```python
from build123d import *

# Parameters (mm, degrees)
F2_DEPTH   = 3.175
F1_R       = 3.3099800026
F2_FACE_R  = 15.875
F3_DEPTH   = 3.176
F4_DEPTH   = 3.176
F5_DEPTH   = 3.176
F1_W       = 6.5204764251
F1_H       = 1.0553477332
F6_DEPTH   = 3.429
F7_DEPTH   = 3.175
F8_DEPTH   = 3.175
F10_DEPTH  = 3.175
F1_R_2     = 1.2371702014
F10_FACE_R = 3.3099800026
F10_FACE_W = 6.5204764251
F10_FACE_H = 1.0553477332
F11_DEPTH  = 3.43
F12_DEPTH  = 3.429


with BuildPart() as f2:
    # F0 (on Front) → F2 (new body)
    with BuildSketch(Plane.XZ):
        with BuildLine():
            ThreePointArc((-15.3480242567, 4.0563254821), (-2.0452065819, -15.7427048196), (15.875, 0))
            ThreePointArc((15.875, 0), (15.3869963752, 3.9058888297), (13.9529883401, 7.5716406003))
            ThreePointArc((13.9529883401, 7.5716406003), (12.6412349384, 9.6028539629), (11.0362168136, 11.4112901743))
            ThreePointArc((11.0362168136, 11.4112901743), (9.0476421038, 13.0443779983), (6.8213515593, 14.3347405943))
            ThreePointArc((6.8213515593, 14.3347405943), (5.0774604505, 15.0411110086), (3.2622452096, 15.5361958404))
            ThreePointArc((3.2622452096, 15.5361958404), (1.6398957334, 15.7900717853), (0, 15.875))
            ThreePointArc((0, 15.875), (-2.3954258199, 15.693232941), (-4.7359968989, 15.152094191))
            ThreePointArc((-4.7359968989, 15.152094191), (-6.342661706, 14.552878323), (-7.8753225223, 13.7838644861))
            ThreePointArc((-7.8753225223, 13.7838644861), (-9.4847902105, 12.730058117), (-10.9549720741, 11.4893085891))
            ThreePointArc((-10.9549720741, 11.4893085891), (-13.6665362642, 8.0772155808), (-15.3480242567, 4.0563254821))
        make_face()
    extrude(amount=F2_DEPTH)

    # F1 (on face) + F2_face (on face) → F3 (cut, through all)
    with BuildSketch(Plane.XZ):
        with Locations((-6.1555983319, 4.3306481437)):
            Circle(F1_R)
    with BuildSketch(Plane.XZ.offset(3.175)):
        Circle(F2_FACE_R)
    extrude(amount=F3_DEPTH, mode=Mode.SUBTRACT)

    # F1 (on face) → F4 (cut, through all)
    with BuildSketch(Plane.XZ):
        with Locations((6.1544640741, 4.4018082744)):
            Circle(F1_R)
    extrude(amount=F4_DEPTH, mode=Mode.SUBTRACT)

    # F1 (on face) → F5 (cut, through all)
    with BuildSketch(Plane.XZ):
        with BuildLine():
            Line((13.2357986914, 0.0787362223), (-13.2809156822, 0.0787362223))
            ThreePointArc((-13.2809156822, 0.0787362223), (-0.0225584954, -11.1437029045), (13.2357986914, 0.0787362223))
        make_face()
    extrude(amount=F5_DEPTH, mode=Mode.SUBTRACT)

    # F1 (on face) → F6 (join)
    with BuildSketch(Plane.XZ):
        with Locations((6.1458884738, 9.15713422)):
            Rectangle(F1_W, F1_H)
    extrude(amount=F6_DEPTH)

    # F0 (on Front) → F7 (join)
    with BuildSketch(Plane.XZ):
        with BuildLine():
            Line((-11.9195533916, 18.9222916961), (-15.3480242567, 4.0563254821))
            ThreePointArc((-15.3480242567, 4.0563254821), (-13.6665362642, 8.0772155808), (-10.9549720741, 11.4893085891))
            Line((-10.9549720741, 11.4893085891), (-11.9195533916, 18.9222916961))
        make_face()
    extrude(amount=F7_DEPTH)

    # F0 (on Front) → F8 (join)
    with BuildSketch(Plane.XZ):
        with BuildLine():
            Line((-7.8753225223, 24.8427737317), (-10.9549720741, 11.4893085891))
            ThreePointArc((-10.9549720741, 11.4893085891), (-9.4847902105, 12.730058117), (-7.8753225223, 13.7838644861))
            Line((-7.8753225223, 13.7838644861), (-7.8753225223, 24.8427737317))
        make_face()
    extrude(amount=F8_DEPTH)

    # F0 (on Front) → F10 (join)
    with BuildSketch(Plane.XZ):
        with BuildLine():
            Line((0, 29.9478769302), (-4.7359968989, 15.152094191))
            ThreePointArc((-4.7359968989, 15.152094191), (-2.3954258199, 15.693232941), (0, 15.875))
            Line((0, 15.875), (0, 29.9478769302))
        make_face()
        with BuildLine():
            ThreePointArc((0, 15.875), (1.6398957334, 15.7900717853), (3.2622452096, 15.5361958404))
            Line((3.2622452096, 15.5361958404), (3.2622452096, 30.0202061216))
            Line((3.2622452096, 30.0202061216), (0, 15.875))
        make_face()
        with BuildLine():
            ThreePointArc((3.2622452096, 15.5361958404), (5.0774604505, 15.0411110086), (6.8213515593, 14.3347405943))
            Line((6.8213515593, 14.3347405943), (9.8336311057, 27.3960871034))
            Line((9.8336311057, 27.3960871034), (3.2622452096, 15.5361958404))
        make_face()
        with BuildLine():
            ThreePointArc((6.8213515593, 14.3347405943), (9.0476421038, 13.0443779983), (11.0362168136, 11.4112901743))
            Line((11.0362168136, 11.4112901743), (14.0054738149, 24.286089465))
            Line((14.0054738149, 24.286089465), (6.8213515593, 14.3347405943))
        make_face()
        with BuildLine():
            ThreePointArc((11.0362168136, 11.4112901743), (12.6412349384, 9.6028539629), (13.9529883401, 7.5716406003))
            Line((13.9529883401, 7.5716406003), (17.5813417882, 19.8162570596))
            Line((17.5813417882, 19.8162570596), (11.0362168136, 11.4112901743))
        make_face()
        with BuildLine():
            Line((-4.7359968989, 27.3960871034), (-7.8753225223, 13.7838644861))
            ThreePointArc((-7.8753225223, 13.7838644861), (-6.342661706, 14.552878323), (-4.7359968989, 15.152094191))
            Line((-4.7359968989, 15.152094191), (-4.7359968989, 27.3960871034))
        make_face()
    extrude(amount=F10_DEPTH)

    # F1 (on face) + F10_face (on face) → F11 (cut, through all)
    with BuildSketch(Plane.XZ):
        with Locations((-12.1244213607, 7.7306859973)):
            Circle(F1_R_2)
    with BuildSketch(Plane(origin=(0.4916351087, -3.175, 5.8381828157), x_dir=(1, 0, 0), z_dir=(0, -1, 0))):
        with BuildLine():
            ThreePointArc((-15.8396593653, -1.7818573336), (-2.5368416906, -21.5808876353), (15.3833648913, -5.8381828157))
            ThreePointArc((15.3833648913, -5.8381828157), (14.8953612665, -1.932293986), (13.4613532315, 1.7334577846))
            Line((13.4613532315, 1.7334577846), (17.0897066795, 13.9780742439))
            Line((17.0897066795, 13.9780742439), (10.544581705, 5.5731073586))
            Line((10.544581705, 5.5731073586), (13.5138387063, 18.4479066493))
            Line((13.5138387063, 18.4479066493), (6.3297164506, 8.4965577786))
            Line((6.3297164506, 8.4965577786), (9.3419959971, 21.5579042877))
            Line((9.3419959971, 21.5579042877), (2.770610101, 9.6980130247))
            Line((2.770610101, 9.6980130247), (2.770610101, 24.1820233059))
            Line((2.770610101, 24.1820233059), (-0.4916351087, 10.0368171843))
            Line((-0.4916351087, 10.0368171843), (-0.4916351087, 24.1096941145))
            Line((-0.4916351087, 24.1096941145), (-5.2276320076, 9.3139113753))
            Line((-5.2276320076, 9.3139113753), (-5.2276320076, 21.5579042877))
            Line((-5.2276320076, 21.5579042877), (-8.3669576309, 7.9456816704))
            Line((-8.3669576309, 7.9456816704), (-8.3669576309, 19.004590916))
            Line((-8.3669576309, 19.004590916), (-11.4466071828, 5.6511257734))
            Line((-11.4466071828, 5.6511257734), (-12.4111885003, 13.0841088804))
            Line((-12.4111885003, 13.0841088804), (-15.8396593653, -1.7818573336))
        make_face()
        with BuildLine():
            ThreePointArc((12.7441635827, -5.7594465934), (-0.5141936041, -16.9818857202), (-13.7725507908, -5.7594465934))
            Line((-13.7725507908, -5.7594465934), (12.7441635827, -5.7594465934))
        make_face(mode=Mode.SUBTRACT)
        with Locations((-6.6472334405, -1.507534672)):
            Circle(F10_FACE_R, mode=Mode.SUBTRACT)
        with Locations((5.6628289654, -1.4363745413)):
            Circle(F10_FACE_R, mode=Mode.SUBTRACT)
        with Locations((5.6542533652, 3.3189514043)):
            Rectangle(F10_FACE_W, F10_FACE_H, mode=Mode.SUBTRACT)
    extrude(amount=F11_DEPTH, mode=Mode.SUBTRACT)

    # F1 (on face) → F12 (join)
    with BuildSketch(Plane.XZ):
        with Locations((-5.870418041, 10.2435215376)):
            Rectangle(F1_W, F1_H)
    extrude(amount=F12_DEPTH)


solid = f2.part
```
Model file for the job. Use its own axes, mm. A direction names the side the tool comes from. Coordinates: 2 decimals unless noted, no trailing zeros. Loops run counter-clockwise (first coordinate to the right, second up) from the corner with the lowest first, then second, coordinate; pieces in that order, holes last. Notation, with made-up numbers: M 56.5,10 L 92.5,10 A25 ccw 92.5,23 Z; hole C 79.25,37 d8. An arc over 180 degrees is marked long. Use CSV: the item, a comma, the result in double quotes. Start each with the question number.
1. Tool access for faces 4 (the flat face through (10.464, -1.565, 19.38)), 5 (the flat face through (-2.335, -1.565, 22.654)), 6 (the flat face through (-13.61, -1.57, 11.59)): list every direction of +Z, -Z, +X, -X, +Y, -Y with a clear straight run to the whole face (end or side of a thin tool).
2. Probe probe 1 along X at (y, z) = (-1.1, 1.5); probe 2 along X at (y, z) = (-2.05, 5.5); probe 3 along Z at (x, y) = (4, -0.25). List the from-to ranges inside material, lowest first. Write a range as [from, to].
3. Band-saw the part on B-B, the plane x = 2. List the corners of the cut face in (y, z) (3 decimals), then the cut area to 3 significant figures.
4. Band-saw the part on D-D, the plane y = -1.45. List the corners of the cut face in (x, z) (3 decimals), then the cut area to 3 significant figures.
5. Two-plate mould, pull along Z, no slides. Class faces 1 (the flat face through (3.262, -2, 23)), 2 (the flat face through (15.742, -1.565, 13.608)), 3 (the flat face through (-9.394, -1.565, 18.26)): pulls with the +Z half, pulls with the -Z half, needs draft (parallel to the pull), parting line crosses it, or undercut.
6. Band-saw the part on A-A, the plane z = -7.5. List the corners of the cut face in (x, y) (3 decimals), then the cut area to 3 significant figures.
7. Flat gauge pins, fed straight in: pin 1 (1.6 mm diameter, centred on y = -1.5, z = 19, fed in from +X); pin 2 (1 mm diameter, centred on y = -2.5, z = 19, fed in from +X); pin 3 (7.5 mm diameter, centred on x = -6.16, z = 4.33, fed in from -Y) (3 decimals). Where does each tip first touch, or does it go through?
8. Band-saw the part on C-C, the plane z = 5. List the corners of the cut face in (x, y) (3 decimals), then the cut area to 3 significant figures.
Entries:
1,face 4,"+Y, -Y"
1,face 5,"+Z, +Y, -Y"
1,face 6,"+Z, -X, +Y, -Y"
2,probe 1,"x = [-15.8, -7.87], [-4.44, 4.56], [7.75, 15.8]"
2,probe 2,"x = [-15.02, -9.25], [-3.06, 3.03], [9.28, 14.89]"
2,probe 3,"z = [-15.36, -10.53], [0.08, 1.89], [6.91, 16.87]"
3,outline,"M -3.175,-15.749 L 0,-15.749 L 0,-10.991 L -3.175,-10.991 Z; M -3.175,0.079 L 0,0.079 L 0,24.547 L -3.175,24.547 Z"
3,area,"92.8 mm2"
4,outline,"M -15.348,4.056 A15.875 ccw long 13.953,7.572 L 17.581,19.816 L 11.036,11.411 L 14.005,24.286 L 6.821,14.335 L 9.834,27.396 L 3.262,15.536 L 3.262,30.02 L 0,15.875 L 0,29.948 L -4.736,15.152 L -4.736,27.396 L -7.875,13.784 L -7.875,24.843 L -10.955,11.489 L -11.92,18.922 Z; hole C -12.124,7.731 d2.474; hole M -13.281,0.079 A13.443 ccw 13.236,0.079 Z; hole C -6.156,4.331 d6.62; hole C 6.154,4.402 d6.62"
4,area,"682 mm2"
5,face 1,"needs draft"
5,face 2,"undercut"
5,face 3,"pulls with the +Z half"
6,outline,"M -13.992,-3.175 L -9.225,-3.175 L -9.225,0 L -13.992,0 Z; M 9.18,-3.175 L 13.992,-3.175 L 13.992,0 L 9.18,0 Z"
6,area,"30.4 mm2"
7,pin 1,"stops at x = 17.58"
7,pin 2,"stops at x = 17.49"
7,pin 3,"stops at y = -3.175"
8,outline,"M -15.13,-3.175 L -9.397,-3.175 L -9.397,0 L -15.13,0 Z; M -2.914,-3.175 L 2.899,-3.175 L 2.899,0 L -2.914,0 Z; M 9.41,-3.175 L 15.067,-3.175 L 15.067,0 L 9.41,0 Z"
8,area,"54.6 mm2"
